```python
from build123d import *

# Parameters (mm, degrees)
F2_R     = 11
F2_R_2   = 10
F2_R_3   = 8
F2_R_4   = 7
F2_R_5   = 5
F2_R_6   = 4
F3_DEPTH = 1
F4_SIZE  = 0.4
F5_SIZE  = 0.4


with BuildPart() as f1:
    # F0 (on Front) → F1 (revolve)
    with BuildSketch(Plane.XZ):
        with BuildLine():
            Line((0, 12.75), (0, 0))
            Line((0, 0), (13, 0))
            ThreePointArc((13, 0), (16.535534, 1.464466), (18, 5))
            Line((18, 5), (18, 35))
            Line((18, 35), (6.1, 35))
            Line((6.1, 35), (4.6, 32.5))
            Line((4.6, 32.5), (4.6, 12.75))
            Line((4.6, 12.75), (0, 12.75))
        make_face()
    revolve(axis=Axis((0, 0, 24.334948), (0, 0, 1)))

    # F2 (on face) → F3 (cut)
    with BuildSketch(Plane(origin=(0, 0, 0), x_dir=(1, 0, 0), z_dir=(0, 0, -1))):
        Circle(F2_R)
        Circle(F2_R_2, mode=Mode.SUBTRACT)
        Circle(F2_R_3)
        Circle(F2_R_4, mode=Mode.SUBTRACT)
        Circle(F2_R_5)
        Circle(F2_R_6, mode=Mode.SUBTRACT)
    extrude(amount=-F3_DEPTH, mode=Mode.SUBTRACT)

    # F4
    f4_edges = [f1.edges().sort_by_distance(p)[0] for p in [
        (-11, 0, 0),
        (-10, 0, 0),
        (-8, 0, 0),
        (-7, 0, 0),
        (-5, 0, 0),
        (-4, 0, 0),
    ]]
    chamfer(f4_edges, length=F4_SIZE)

    # F5
    f5_edges = [f1.edges().sort_by_distance(p)[0] for p in [
        (-11, 0, 1),
        (-10, 0, 1),
        (-8, 0, 1),
        (-7, 0, 1),
        (-5, 0, 1),
        (-4, 0, 1),
    ]]
    chamfer(f5_edges, length=F5_SIZE)


solid = f1.part
```
Input: part model. Units: mm. Frame: model coordinates. Round coordinates to 2 decimals unless told otherwise and drop trailing zeros. Order: outer loops, then holes, each group sorted by start corner. A loop starts at its lowest first (then second) coordinate and runs counter-clockwise, first axis right, second up. Notation, with made-up numbers: (4.25, 8) - (10.25, 8) arc R20 cw to (10.25, 34) - close; hole circle Ø11 at (-28.5, 12.5). An arc over 180 degrees is marked (long way). One line per question, with ' | ' between items. Start each with the question number.
1) Cut plane B-B, the plane z = 9. Return the cut outline in (x, y).
2) Contact query for flat-ended pins moving along their axis: P1, Ø7.5, axis at x = 2, y = 2.5, coming from the -Z side; P2, Ø7.5, axis at x = 0, y = 0, coming from the +Z side; P3, Ø10, axis at y = 13, z = 12.5, coming from the +X side; P4, Ø8, axis at x = -3, z = 4, coming from the -Y side. Output: stop coordinate, or through.
3) Ray query, probe 1 along Y at (x, z) = (0, 23.5); probe 2 along X at (y, z) = (-1, 15.5); probe 3 along Z at (x, y) = (1, -3). Return the intervals inside material, ascending.
4) Cut plane A-A, the plane z = 13.5. Return the cut outline in (x, y), then the cut area to 3 significant figures.
Worked out:
1) outline: circle Ø36 at (0, 0)
2) P1: stops at z = 0 | P2: stops at z = 12.75 | P3: stops at x = 16.12 | P4: stops at y = -18
3) probe 1: y = -18 to -4.6, 4.6 to 18 | probe 2: x = -17.97 to -4.49, 4.49 to 17.97 | probe 3: z = 0 to 12.75
4) outline: circle Ø36 at (0, 0); hole circle Ø9.2 at (0, 0) | area: 951 mm^2
